```python
from build123d import *

# Parameters (mm, degrees)
F1_DEPTH = 19.05


with BuildPart() as f1:
    # F0 (on Front) → F1 (new body)
    with BuildSketch(Plane.XZ):
        Polygon((-80.3030704341, -65.7893445744), (-180.6575025499, -65.7893445744), (-180.6575025499, -84.8393445744), (-80.3030704341, -84.8393445744), (-47.3075025499, -84.8393445744), (-47.3075025499, -75.3143445744), (-47.3075025499, -65.7893445744), align=None)
        Polygon((-47.3075025499, -46.7393445744), (-80.3030704341, -65.7893445744), (-47.3075025499, -65.7893445744), align=None)
        Polygon((-47.3075025499, -46.7393445744), (-47.3075025499, -65.7893445744), (-40.9575025499, -65.7893445744), (-34.6075025499, -65.7893445744), (-34.6075025499, -46.7393445744), align=None)
        with BuildLine():
            Line((-40.9575025499, -65.7893445744), (-47.3075025499, -65.7893445744))
            Line((-47.3075025499, -65.7893445744), (-47.3075025499, -75.3143445744))
            ThreePointArc((-47.3075025499, -75.3143445744), (-45.4476306104, -70.8242165139), (-40.9575025499, -68.9643445744))
            Line((-40.9575025499, -68.9643445744), (-40.9575025499, -65.7893445744))
        make_face()
        Polygon((-47.3075025499, -84.8393445744), (-80.3030704341, -84.8393445744), (-47.3075025499, -103.8893445744), align=None)
        with BuildLine():
            Line((-34.6075025499, -65.7893445744), (-40.9575025499, -65.7893445744))
            Line((-40.9575025499, -65.7893445744), (-40.9575025499, -68.9643445744))
            ThreePointArc((-40.9575025499, -68.9643445744), (-36.4673744894, -70.8242165139), (-34.6075025499, -75.3143445744))
            Line((-34.6075025499, -75.3143445744), (-34.6075025499, -65.7893445744))
        make_face()
        with BuildLine():
            ThreePointArc((-40.9575025499, -81.6643445744), (-45.4476306104, -79.8044726349), (-47.3075025499, -75.3143445744))
            Line((-47.3075025499, -75.3143445744), (-47.3075025499, -84.8393445744))
            Line((-47.3075025499, -84.8393445744), (-43.3831779935, -84.8393445744))
            Line((-43.3831779935, -84.8393445744), (-40.9575025499, -84.8393445744))
            Line((-40.9575025499, -84.8393445744), (-40.9575025499, -81.6643445744))
        make_face()
        Polygon((-2.8575025499, -65.0702156212), (-34.6075025499, -46.7393445744), (-34.6075025499, -65.7893445744), (-4.1030704341, -65.7893445744), align=None)
        Polygon((28.8924974501, -46.7393445744), (-34.6075025499, -46.7393445744), (-2.8575025499, -65.0702156212), align=None)
        Polygon((-43.3831779935, -84.8393445744), (-47.3075025499, -84.8393445744), (-47.3075025499, -103.8893445744), (-34.6075025499, -103.8893445744), (-34.6075025499, -84.8393445744), (-40.9575025499, -84.8393445744), align=None)
        Polygon((-4.1030704341, -65.7893445744), (-34.6075025499, -65.7893445744), (-34.6075025499, -75.3143445744), (-34.6075025499, -84.8393445744), (-4.1030704341, -84.8393445744), (-2.8575025499, -84.8393445744), (-2.8575025499, -65.7893445744), align=None)
        with BuildLine():
            ThreePointArc((-34.6075025499, -75.3143445744), (-36.4673744894, -79.8044726349), (-40.9575025499, -81.6643445744))
            Line((-40.9575025499, -81.6643445744), (-40.9575025499, -84.8393445744))
            Line((-40.9575025499, -84.8393445744), (-34.6075025499, -84.8393445744))
            Line((-34.6075025499, -84.8393445744), (-34.6075025499, -75.3143445744))
        make_face()
        Polygon((28.8924974501, -46.7393445744), (-2.8575025499, -65.0702156212), (-1.6119346657, -65.7893445744), (28.8924974501, -65.7893445744), align=None)
        Polygon((41.5924974501, -46.7393445744), (28.8924974501, -46.7393445744), (28.8924974501, -65.7893445744), (35.2424974501, -65.7893445744), (41.5924974501, -65.7893445744), align=None)
        Polygon((-34.6075025499, -84.8393445744), (-34.6075025499, -103.8893445744), (-2.8575025499, -85.5584735276), (-4.1030704341, -84.8393445744), align=None)
        Polygon((-2.8575025499, -85.5584735276), (-34.6075025499, -103.8893445744), (28.8924974501, -103.8893445744), align=None)
        Polygon((28.8924974501, -65.7893445744), (-1.6119346657, -65.7893445744), (-2.8575025499, -65.7893445744), (-2.8575025499, -84.8393445744), (-1.6119346657, -84.8393445744), (28.8924974501, -84.8393445744), (28.8924974501, -75.3143445744), align=None)
        Polygon((74.5880653343, -65.7893445744), (41.5924974501, -46.7393445744), (41.5924974501, -65.7893445744), align=None)
        with BuildLine():
            Line((35.2424974501, -65.7893445744), (28.8924974501, -65.7893445744))
            Line((28.8924974501, -65.7893445744), (28.8924974501, -75.3143445744))
            ThreePointArc((28.8924974501, -75.3143445744), (30.7523693896, -70.8242165139), (35.2424974501, -68.9643445744))
            Line((35.2424974501, -68.9643445744), (35.2424974501, -65.7893445744))
        make_face()
        Polygon((-1.6119346657, -84.8393445744), (-2.8575025499, -85.5584735276), (28.8924974501, -103.8893445744), (28.8924974501, -84.8393445744), align=None)
        Polygon((28.8924974501, -84.8393445744), (28.8924974501, -103.8893445744), (41.5924974501, -103.8893445744), (41.5924974501, -84.8393445744), (35.2424974501, -84.8393445744), align=None)
        with BuildLine():
            Line((41.5924974501, -75.3143445744), (41.5924974501, -65.7893445744))
            Line((41.5924974501, -65.7893445744), (35.2424974501, -65.7893445744))
            Line((35.2424974501, -65.7893445744), (35.2424974501, -68.9643445744))
            ThreePointArc((35.2424974501, -68.9643445744), (39.7326255106, -70.8242165139), (41.5924974501, -75.3143445744))
        make_face()
        Polygon((74.5880653343, -65.7893445744), (41.5924974501, -65.7893445744), (41.5924974501, -75.3143445744), (41.5924974501, -84.8393445744), (74.5880653343, -84.8393445744), (174.9424974501, -84.8393445744), (174.9424974501, -65.7893445744), align=None)
        with BuildLine():
            ThreePointArc((35.2424974501, -81.6643445744), (30.7523693896, -79.8044726349), (28.8924974501, -75.3143445744))
            Line((28.8924974501, -75.3143445744), (28.8924974501, -84.8393445744))
            Line((28.8924974501, -84.8393445744), (35.2424974501, -84.8393445744))
            Line((35.2424974501, -84.8393445744), (35.2424974501, -81.6643445744))
        make_face()
        Polygon((41.5924974501, -84.8393445744), (41.5924974501, -103.8893445744), (74.5880653343, -84.8393445744), align=None)
        with BuildLine():
            Line((41.5924974501, -84.8393445744), (41.5924974501, -75.3143445744))
            ThreePointArc((41.5924974501, -75.3143445744), (39.7326255106, -79.8044726349), (35.2424974501, -81.6643445744))
            Line((35.2424974501, -81.6643445744), (35.2424974501, -84.8393445744))
            Line((35.2424974501, -84.8393445744), (41.5924974501, -84.8393445744))
        make_face()
    extrude(amount=F1_DEPTH)


solid = f1.part
```
Geometry check sheet. Reference: the model listing, model coordinates, mm. A direction names the side the tool comes from. Coordinates: 2 decimals unless noted, no trailing zeros. Loops run counter-clockwise (first coordinate to the right, second up) from the corner with the lowest first, then second, coordinate; pieces in that order, holes last.
Item 1: Go/stop test with flat-tipped pins: pin 1 Ø9.5 at (x, y) = (-125.5, -12.5) entering from +Z; pin 2 Ø4 at (x, y) = (71.5, -14) entering from +Z; pin 3 Ø5.5 at (x, y) = (128.5, -6.5) entering from -Z. Record where each tip stops, or that it passes through.
Item 2: Sectioned sample at D-D, the plane x = 104. Record the boundary of the cut face in (y, z), then the cut area to 3 significant figures.
Item 3: Thickness scan on line 1 (X direction, y = -7, z = -79); line 2 (X direction, y = -12, z = -73.5); line 3 (Z direction, x = 105.5, y = -4.5). Record the ranges inside material, lowest first.
Item 4: Access from +Z, -Z, +X, -X, +Y, -Y to the whole of each face (thin tool, end or side, straight path). Record for faces 1 (the face through (125, -9, -65.789)), 2 (the face through (124, -9, -84.839)), 3 (the face through (-130, -9, -65.789)).
Item 5: Sectioned sample at A-A, the plane y = -3.75. Record the boundary of the cut face in (x, z).
Item 6: Sectioned sample at B-B, the plane x = 38.5. Record the boundary of the cut face in (y, z), then the cut area to 3 significant figures.
Item 7: Sectioned sample at C-C, the plane z = -59.5. Record the boundary of the cut face in (x, y).
Check result:
1. pin 1: stops at z = -65.79
1. pin 2: stops at z = -62.85
1. pin 3: stops at z = -84.84
2. outline: (-19.05, -84.84) - (0, -84.84) - (0, -65.79) - (-19.05, -65.79) - close
2. area: 363 mm2
3. line 1: x = -180.66 to -46.13, -35.79 to 30.07, 40.41 to 174.94
3. line 2: x = -180.66 to -47.04, -34.87 to 29.16, 41.33 to 174.94
3. line 3: z = -84.84 to -65.79
4. face 1: +Z, +X, +Y, -Y
4. face 2: -Z, +X, +Y, -Y
4. face 3: +Z, -X, +Y, -Y
5. outline: (-180.66, -84.84) - (-80.3, -84.84) - (-47.31, -103.89) - (41.59, -103.89) - (74.59, -84.84) - (174.94, -84.84) - (174.94, -65.79) - (74.59, -65.79) - (41.59, -46.74) - (-47.31, -46.74) - (-80.3, -65.79) - (-180.66, -65.79) - close; hole circle Ø12.7 at (-40.96, -75.31); hole (-4.1, -84.84) - (-2.86, -85.56) - (-1.61, -84.84) - close; hole (-4.1, -65.79) - (-1.61, -65.79) - (-2.86, -65.07) - close; hole circle Ø12.7 at (35.24, -75.31)
6. outline: (-19.05, -103.89) - (0, -103.89) - (0, -80.77) - (-19.05, -80.77) - close; (-19.05, -69.86) - (0, -69.86) - (0, -46.74) - (-19.05, -46.74) - close
6. area: 881 mm2
7. outline: (-69.41, -19.05) - (63.69, -19.05) - (63.69, 0) - (-69.41, 0) - close
